```python
from build123d import *

# Parameters (mm, degrees)
F0_R     = 1.9939
F1_DEPTH = 63.5
F2_R     = 12.7
F3_DEPTH = 19.05
F4_R     = 22.225
F5_DEPTH = 3.175
F6_R     = 15.875
F7_DEPTH = 3.175


with BuildPart() as f1:
    # F0 (on Top) → F1 (new body)
    with BuildSketch(Plane.XY):
        with BuildLine():
            ThreePointArc((-25.4, -33.1), (-23.935534, -36.635534), (-20.4, -38.1))
            Line((-20.4, -38.1), (20.4, -38.1))
            ThreePointArc((20.4, -38.1), (23.935534, -36.635534), (25.4, -33.1))
            Line((25.4, -33.1), (25.4, 33.1))
            ThreePointArc((25.4, 33.1), (23.935534, 36.635534), (20.4, 38.1))
            Line((20.4, 38.1), (-20.4, 38.1))
            ThreePointArc((-20.4, 38.1), (-23.935534, 36.635534), (-25.4, 33.1))
            Line((-25.4, 33.1), (-25.4, -33.1))
        make_face()
        with Locations((-20.4, -33.1)):
            Circle(F0_R, mode=Mode.SUBTRACT)
        with Locations((20.4, -33.1)):
            Circle(F0_R, mode=Mode.SUBTRACT)
        with Locations((-20.4, 33.1)):
            Circle(F0_R, mode=Mode.SUBTRACT)
        with Locations((20.4, 33.1)):
            Circle(F0_R, mode=Mode.SUBTRACT)
    extrude(amount=F1_DEPTH)

    # F2 (on face) → F3 (join)
    with BuildSketch(Plane(origin=(0, 0, 0), x_dir=(1, 0, 0), z_dir=(0, 0, -1))):
        Circle(F2_R)
    extrude(amount=F3_DEPTH)

    # F4 (on face) → F5 (join)
    with BuildSketch(Plane(origin=(0, 0, 0), x_dir=(1, 0, 0), z_dir=(0, 0, -1))):
        Circle(F4_R)
    extrude(amount=F5_DEPTH)

    # F6 (on face) → F7 (join)
    with BuildSketch(Plane(origin=(0, 0, -19.05), x_dir=(1, 0, 0), z_dir=(0, 0, -1))):
        Circle(F6_R)
    extrude(amount=F7_DEPTH)


solid = f1.part
```
Input: part model. Units: mm. Frame: model coordinates. A direction names the side the tool comes from. Give positions to 0.01 mm unless a question says otherwise; leave off trailing zeros. Order: outer loops, then holes, each group sorted by start corner. A loop starts at its lowest first (then second) coordinate and runs counter-clockwise, first axis right, second up. Notation, with made-up numbers: (12.5, 69) - (17.5, 69) arc R22 ccw to (17.5, 87) - close; hole circle Ø6 at (40, 12). An arc over 180 degrees is marked (long way). Put each result on its own line as item: value.
Item 1: Section query A-A, the plane z = 35. Return loops of the section in (x, y), then the cut area to 3 significant figures.
Found:
outline: (-25.4, -33.1) arc R5 ccw to (-20.4, -38.1) - (20.4, -38.1) arc R5 ccw to (25.4, -33.1) - (25.4, 33.1) arc R5 ccw to (20.4, 38.1) - (-20.4, 38.1) arc R5 ccw to (-25.4, 33.1) - close; hole circle Ø3.99 at (-20.4, -33.1); hole circle Ø3.99 at (-20.4, 33.1); hole circle Ø3.99 at (20.4, -33.1); hole circle Ø3.99 at (20.4, 33.1)
area: 3,800 mm^2
Item 2: Draft query along Z for faces 1 (the flat face through (0, 1, 63.5)), 2 (the flat face through (-7, -11, -19.05)), 3 (the flat face through (-25.4, 0, 31)). Return one class per face: +Z half, -Z half, draft (parallel to the pull), parting line (faces both ways), or undercut.
Found:
face 1: +Z half
face 2: undercut
face 3: draft
Item 3: Section query C-C, the plane x = 0. Return loops of the section in (y, z) (3 decimals), then the cut area to 3 significant figures.
Found:
outline: (-38.1, 0) - (-22.225, 0) - (-22.225, -3.175) - (-12.7, -3.175) - (-12.7, -19.05) - (-15.875, -19.05) - (-15.875, -22.225) - (15.875, -22.225) - (15.875, -19.05) - (12.7, -19.05) - (12.7, -3.175) - (22.225, -3.175) - (22.225, 0) - (38.1, 0) - (38.1, 63.5) - (-38.1, 63.5) - close
area: 5,480 mm^2
Item 4: Ray query, L1, parallel to Y at x = 20.4, z = 22; L2, parallel to Z at x = 9.5, y = -10 (3 decimals); L3, parallel to Z at x = -1, y = -24. Return the intervals inside material, ascending. Write a range as from..to.
Found:
L1: y = -38.1..-35.09, -31.11..31.11, 35.09..38.1
L2: z = -22.225..-19.05, -3.175..63.5
L3: z = 0..63.5
Item 5: Access query for faces 4 (the cylindrical face through (-3.441, 15.497, -20.615)), 5 (the cylindrical face through (-20.66, -31.123, 31.306)), 6 (the flat face through (10, 10, -3.175)). Directions: +Z, -Z, +X, -X, +Y, -Y. A direction counts if a zero-diameter tool reaches every point of the face in a straight line with its end or side. Return the directions, or none.
Found:
face 4: -Z
face 5: +Z, -Z
face 6: none
Item 6: Section query B-B, the plane y = 0. Return loops of the section in (x, z) (3 decimals).
Found:
outline: (-25.4, 0) - (-22.225, 0) - (-22.225, -3.175) - (-12.7, -3.175) - (-12.7, -19.05) - (-15.875, -19.05) - (-15.875, -22.225) - (15.875, -22.225) - (15.875, -19.05) - (12.7, -19.05) - (12.7, -3.175) - (22.225, -3.175) - (22.225, 0) - (25.4, 0) - (25.4, 63.5) - (-25.4, 63.5) - close
Item 7: Section query D-D, the plane z = -6. Return loops of the section in (x, y).
Found:
outline: circle Ø25.4 at (0, 0)
Item 8: Contact query for flat-ended pins moving along their axis: pin 1 (5 mm diameter, centred on x = 13, z = -3.5, fed in from -Y); pin 2 (5 mm diameter, centred on x = 20.4, y = -33.1, fed in from -Z); pin 3 (6.5 mm diameter, centred on x = -20.4, y = -33.1, fed in from +Z); pin 4 (1.5 mm diameter, centred on x = 11, y = -19, fed in from -Z) (3 decimals). Output: stop coordinate, or through.
Found:
pin 1: stops at y = -19.58
pin 2: stops at z = 0
pin 3: stops at z = 63.5
pin 4: stops at z = -3.175
